Build history of the part. All positions in model axes, mm. Round coordinates to 2 decimals unless told otherwise and drop trailing zeros. Write each loop counter-clockwise with the first axis right and the second up, starting at its lowest first coordinate (ties: lowest second). Pieces come first, ordered by that corner, then holes. Notation, with made-up numbers: (-23.5, 73.25) - (22.5, 73.25) arc R18 ccw to (22.5, 103.25) - close; hole circle Ø10 at (36.25, 1.5). An arc over 180 degrees is marked (long way). Answer as a JSON object with one key per item and string values. Group by question number.
Item 1: Slice it at A-A, the plane x = 0. List the corners of the cut face in (y, z) (3 decimals), then the cut area to 3 significant figures.
Item 2: Slice it at C-C, the plane x = -10.25. List the corners of the cut face in (y, z), then the cut area to 3 significant figures.
Item 3: Flat gauge pins, fed straight in: pin 1 (2.5 mm diameter, centred on y = -3, z = -6.5, fed in from +X); pin 2 (7.5 mm diameter, centred on x = 0, z = -3, fed in from +Y); pin 3 (1.6 mm diameter, centred on y = -3.5, z = 5.5, fed in from +X); pin 4 (4 mm diameter, centred on x = 0, z = 0, fed in from -Y). Where does each tip first touch, or does it go through?
Item 4: Probe line 1 (Z direction, x = -10.5, y = 8.75); line 2 (Z direction, x = 0, y = 9.1) (3 decimals); line 3 (Z direction, x = 0, y = 3.75). List the from-to ranges inside material, lowest first. Write a range as from..to.
Item 5: Slice it at B-B, the plane z = 0. List the corners of the cut face in (x, y) (3 decimals).
Item 6: Slice it at D-D, the plane y = 3. List the corners of the cut face in (x, z), then the cut area to 3 significant figures.
Autodesk Inventor part; units mm, degrees
ref_plane "YZ Plane" through (0, 0, 0) normal (1, 0, 0) x (0, 1, 0)
ref_plane "XZ Plane" through (0, 0, 0) normal (0, 1, 0) x (-1, 0, 0)
ref_plane "XY Plane" through (0, 0, 0) normal (0, 0, 1) x (1, 0, 0)
sketch "Sketch1" plane through (0, 0, 0) normal (0, 1, 0) x (-1, 0, 0)
  line L0 (30, 48) -> (-30, 48)
  line L1 (-30, 48) -> (-30, -48)
  line L2 (-30, -48) -> (30, -48)
  line L3 (30, -48) -> (30, 48)
  line L4 (30, 48) -> (-30, -48) construction
  line L5 (-30, 48) -> (30, -48) construction
  point P0 (0, 0)
  dimension "d0" = 60
  dimension "d1" = 96
extrude "Extrusion1" add sketch "Sketch1" along normal blind 10
sketch "Sketch2" plane through (0, 10, 0) normal (0, 1, 0) x (1, 0, 0)
  line L0 (13, -30.5) -> (13, 30.5) construction
  line L1 (13, 30.5) -> (-13, 30.5) construction
  line L2 (-13, 30.5) -> (-13, -30.5) construction
  line L3 (-13, -30.5) -> (13, -30.5) construction
  line L4 (13, -30.5) -> (-13, 30.5) construction
  line L5 (13, 30.5) -> (-13, -30.5) construction
  line L6 (-13, -30.5) -> (-10.25, -30.5)
  line L7 (-13, 30.5) -> (-10.25, 30.5)
  line L8 (13, -30.5) -> (10.25, -30.5) construction
  line L9 (13, 30.5) -> (10.25, 30.5)
  line L10 (10.25, -36.5) -> (10.25, -24.5) construction
  line L11 (13, -36.5) -> (13, -24.5)
  line L12 (7.5, -24.5) -> (7.5, -36.5)
  arc A0 (7.5, -36.5) -> (13, -36.5) centre (10.25, -36.5) ccw
  arc A1 (13, -24.5) -> (7.5, -24.5) centre (10.25, -24.5) ccw
  arc A2 (-13, -36.5) -> (-7.5, -36.5) centre (-10.25, -36.5) ccw
  line L13 (-13, -24.5) -> (-13, -36.5)
  line L14 (-7.5, -36.5) -> (-7.5, -24.5)
  arc A3 (-7.5, -24.5) -> (-13, -24.5) centre (-10.25, -24.5) ccw
  arc A4 (7.5, 24.5) -> (13, 24.5) centre (10.25, 24.5) ccw
  line L15 (7.5, 36.5) -> (7.5, 24.5)
  line L16 (13, 24.5) -> (13, 36.5)
  arc A5 (13, 36.5) -> (7.5, 36.5) centre (10.25, 36.5) ccw
  arc A6 (-13, 24.5) -> (-7.5, 24.5) centre (-10.25, 24.5) ccw
  line L17 (-13, 36.5) -> (-13, 24.5)
  line L18 (-7.5, 24.5) -> (-7.5, 36.5)
  arc A7 (-7.5, 36.5) -> (-13, 36.5) centre (-10.25, 36.5) ccw
  point P0 (0, 0)
  point P1 (0, 0)
  point P2 (0, 0)
  dimension "d17" = 61
  dimension "d16" = 26
  dimension "d13" = 2.75
  dimension "d15" = 2.75
  dimension "d12" = 2.75
  dimension "d14" = 2.75
  dimension "d11" = 6
  dimension "d10" = 5.5
  dimension "d8" = 6
  dimension "d9" = 5.5
  dimension "d6" = 6
  dimension "d7" = 5.5
  dimension "d4" = 6
  dimension "d5" = 5.5
extrude "Extrusion2" cut sketch "Sketch2" against normal through all
sketch "Sketch3" plane through (0, 0, 0) normal (0, -1, 0) x (1, 0, 0)
  circle A0 centre (0, 0) radius 7.275
  line L0 (7.275, 0) -> (-7.275, 0) construction
  line L1 (0, 7.275) -> (0, -7.275) construction
  line L2 (9.775, 2.5) -> (4.775, 2.5)
  line L3 (4.775, 2.5) -> (4.775, -2.5)
  line L4 (4.775, -2.5) -> (9.775, -2.5)
  line L5 (9.775, -2.5) -> (9.775, 2.5)
  line L6 (9.775, 2.5) -> (4.775, -2.5) construction
  line L7 (4.775, 2.5) -> (9.775, -2.5) construction
  line L8 (2.5, 9.775) -> (-2.5, 9.775)
  line L9 (-2.5, 9.775) -> (-2.5, 4.775)
  line L10 (-2.5, 4.775) -> (2.5, 4.775)
  line L11 (2.5, 4.775) -> (2.5, 9.775)
  line L12 (2.5, 9.775) -> (-2.5, 4.775) construction
  line L13 (-2.5, 9.775) -> (2.5, 4.775) construction
  line L14 (-9.775, 2.5) -> (-4.775, 2.5)
  line L15 (-4.775, 2.5) -> (-4.775, -2.5)
  line L16 (-4.775, -2.5) -> (-9.775, -2.5)
  line L17 (-9.775, -2.5) -> (-9.775, 2.5)
  line L18 (-9.775, 2.5) -> (-4.775, -2.5) construction
  line L19 (-4.775, 2.5) -> (-9.775, -2.5) construction
  line L20 (-2.5, -4.775) -> (2.5, -4.775)
  line L21 (2.5, -4.775) -> (2.5, -9.775)
  line L22 (2.5, -9.775) -> (-2.5, -9.775)
  line L23 (-2.5, -9.775) -> (-2.5, -4.775)
  line L24 (-2.5, -4.775) -> (2.5, -9.775) construction
  line L25 (2.5, -4.775) -> (-2.5, -9.775) construction
  point P0 (6.832, 2.5)
  point P1 (2.5, 6.832)
  point P2 (-2.5, 6.832)
  point P3 (-6.832, 2.5)
  point P4 (-6.832, -2.5)
  point P5 (-2.5, -6.832)
  point P6 (2.5, -6.832)
  point P7 (6.832, -2.5)
  dimension "d29" = 14.55
  dimension "d27" = 5
  dimension "d28" = 5
  dimension "d25" = 5
  dimension "d26" = 5
  dimension "d23" = 5
  dimension "d24" = 5
  dimension "d21" = 5
  dimension "d22" = 5
extrude "Extrusion3" add sketch "Sketch3" along normal blind 5 contours L2 L3 L4 A0 L21 L20 L23 L16 L15 L14 L9 L10 L11
sketch "Sketch4" plane through (0, 10, 0) normal (0, 1, 0) x (1, 0, 0)
  line L0 (13, -30.5) -> (13, 30.5) construction
  line L1 (13, 30.5) -> (-13, 30.5) construction
  line L2 (-13, 30.5) -> (-13, -30.5) construction
  line L3 (-13, -30.5) -> (13, -30.5) construction
  line L4 (13, -30.5) -> (-13, 30.5) construction
  line L5 (13, 30.5) -> (-13, -30.5) construction
  line L6 (-13, -30.5) -> (-10.25, -30.5)
  line L7 (-13, 30.5) -> (-10.25, 30.5)
  line L8 (13, -30.5) -> (10.25, -30.5) construction
  line L9 (13, 30.5) -> (10.25, 30.5)
  line L10 (10.25, -36.5) -> (10.25, -24.5) construction
  line L11 (13, -36.5) -> (13, -24.5)
  line L12 (7.5, -24.5) -> (7.5, -36.5)
  arc A0 (7.5, -36.5) -> (13, -36.5) centre (10.25, -36.5) ccw
  arc A1 (13, -24.5) -> (7.5, -24.5) centre (10.25, -24.5) ccw
  arc A2 (-13, -36.5) -> (-7.5, -36.5) centre (-10.25, -36.5) ccw
  line L13 (-13, -24.5) -> (-13, -36.5)
  line L14 (-7.5, -36.5) -> (-7.5, -24.5)
  arc A3 (-7.5, -24.5) -> (-13, -24.5) centre (-10.25, -24.5) ccw
  arc A4 (7.5, 24.5) -> (13, 24.5) centre (10.25, 24.5) ccw
  line L15 (7.5, 36.5) -> (7.5, 24.5)
  line L16 (13, 24.5) -> (13, 36.5)
  arc A5 (13, 36.5) -> (7.5, 36.5) centre (10.25, 36.5) ccw
  arc A6 (-13, 24.5) -> (-7.5, 24.5) centre (-10.25, 24.5) ccw
  line L17 (-13, 36.5) -> (-13, 24.5)
  line L18 (-7.5, 24.5) -> (-7.5, 36.5)
  arc A7 (-7.5, 36.5) -> (-13, 36.5) centre (-10.25, 36.5) ccw
  point P0 (0, 0)
  point P1 (0, 0)
  dimension "d47" = 61
  dimension "d46" = 26
  dimension "d45" = 2.75
  dimension "d44" = 2.75
  dimension "d43" = 2.75
  dimension "d42" = 2.75
  dimension "d41" = 6
  dimension "d40" = 5.5
  dimension "d38" = 6
  dimension "d39" = 5.5
  dimension "d36" = 6
  dimension "d37" = 5.5
  dimension "d34" = 6
  dimension "d35" = 5.5
hole "Hole1" at (0, 10, 0) direction (0, -1, 0) diameter 6.6 end through all counterbore diameter 14.55 counterbore depth 3
fillet "Fillet1" radius 15 4 edges at (30, 5, 48) (-30, 5, 48) (30, 5, -48) (-30, 5, -48)
properties part number "BaseRotationPlate" material "ABS Plastic"
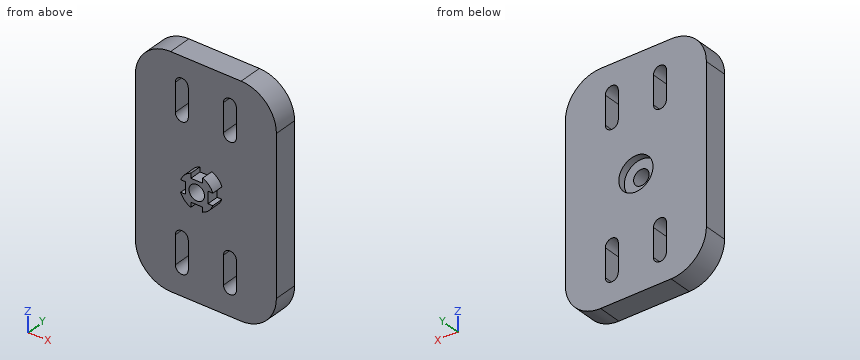
Geometry says:
{
 "1": {"outline": "(-5, -4.775) - (0, -4.775) - (0, -48) - (10, -48) - (10, -7.275) - (7, -7.275) - (7, -3.3) - (-5, -3.3) - close; (-5, 3.3) - (7, 3.3) - (7, 7.275) - (10, 7.275) - (10, 48) - (0, 48) - (0, 4.775) - (-5, 4.775) - close", "area": "885 mm^2"},
 "2": {"outline": "(0, -48) - (10, -48) - (10, -39.25) - (0, -39.25) - close; (0, -21.75) - (10, -21.75) - (10, 21.75) - (0, 21.75) - close; (0, 39.25) - (10, 39.25) - (10, 48) - (0, 48) - close", "area": "610 mm^2"},
 "3": {"pin 1": "stops at x = 5.04", "pin 2": "stops at y = 7", "pin 3": "stops at x = 5.55", "pin 4": "passes through"},
 "4": {"line 1": "z = -48..-39.24, -21.76..21.76, 39.24..48", "line 2": "z = -48..-7.275, 7.275..48", "line 3": "z = -48..-3.3, 3.3..48"},
 "5": {"outline": "(-30, 0) - (-4.775, 0) - (-4.775, -5) - (-3.3, -5) - (-3.3, 7) - (-7.275, 7) - (-7.275, 10) - (-30, 10) - close; (3.3, -5) - (4.775, -5) - (4.775, 0) - (30, 0) - (30, 10) - (7.275, 10) - (7.275, 7) - (3.3, 7) - close"},
 "6": {"outline": "(-30, -33) arc R15 ccw to (-15, -48) - (15, -48) arc R15 ccw to (30, -33) - (30, 33) arc R15 ccw to (15, 48) - (-15, 48) arc R15 ccw to (-30, 33) - close; hole (-13, -36.5) arc R2.75 ccw to (-7.5, -36.5) - (-7.5, -24.5) arc R2.75 ccw to (-13, -24.5) - close; hole (-13, 24.5) arc R2.75 ccw to (-7.5, 24.5) - (-7.5, 36.5) arc R2.75 ccw to (-13, 36.5) - close; hole circle Ø6.6 at (0, 0); hole (7.5, -36.5) arc R2.75 ccw to (13, -36.5) - (13, -24.5) arc R2.75 ccw to (7.5, -24.5) - close; hole (7.5, 24.5) arc R2.75 ccw to (13, 24.5) - (13, 36.5) arc R2.75 ccw to (7.5, 36.5) - close", "area": "5,170 mm^2"}
}
